Read the model definition and answer for the solid it produces. Units are mm, in the model's axes. A direction names the side the tool comes from. Coordinates: 2 decimals unless noted, no trailing zeros. Write each loop counter-clockwise with the first axis right and the second up, starting at its lowest first coordinate (ties: lowest second). Pieces come first, ordered by that corner, then holes.
Item 1: Straight lines are drawn through the part: probe 1 along Z at (x, y) = (-104, -100) (3 decimals); probe 2 along Z at (x, y) = (92, -38.5) (3 decimals); probe 3 along Y at (x, z) = (76.5, 61.5) (3 decimals). For each, find the intervals that lie inside material, in ascending order.
Item 2: Section A-A (x = -60) is taken. Give the vertices of the cut face in (y, z) (3 decimals), then the cut area to 3 significant figures.
Item 3: Section C-C (y = -89) is taken. Give the vertices of the cut face in (x, z) (3 decimals), then the cut area to 3 significant figures.
Item 4: Section B-B (z = 120.5) is taken. Give the vertices of the cut face in (x, y) (3 decimals), then the cut area to 3 significant figures.
Item 5: A tool of negligible diameter and unlimited length cuts with its end or side. For faces 1 (the face through (114.3, -4, 2)), 2 (the face through (-2, 5, 3.175)), from which of +Z, -Z, +X, -X, +Y, -Y can it reach the whole face along a straight path? Write none if from no direction.
Item 6: Determine the mould class of faces 3 (the face through (-101.62, -99.99, 102.13)), 4 (the face through (-102, -100, 27.4)), 5 (the face through (-2, 3, 0)), 6 (the face through (112.39, 99.79, 1.61)) for opening direction Z: released by +Z, released by -Z, zero draft, split by the parting line, or undercut.
Item 7: Each of these flat-tipped pins is pushed along its axis until it touches: P1, Ø8, axis at x = -88.5, y = -28.5, coming from the +Z side (3 decimals); P2, Ø1.5, axis at x = -44, z = 45.5, coming from the +Y side (3 decimals). Where does it stop, or does it pass through?
from build123d import *

# Parameters (mm, degrees)
SKETCH2_W           = 228.6
SKETCH2_H           = 203.2
BOSS_EXTRUDE1_DEPTH = 3.175
SKETCH3_W           = 228.6
SKETCH3_H           = 3.175
BOSS_EXTRUDE2_DEPTH = 127
FILLET1_R           = 3.175
FILLET2_R           = 6.35
SKETCH4_R           = 2.54
SKETCH4_R_2         = 2.15
SKETCH4_R_3         = 3.175
CUT_EXTRUDE1_DEPTH  = 265.612965007


with BuildPart() as part:
    # Sketch2 → Boss-Extrude1 (new body)
    with BuildSketch(Plane.XY):
        Rectangle(SKETCH2_W, SKETCH2_H)
    extrude(amount=BOSS_EXTRUDE1_DEPTH)

    # Sketch3 → Boss-Extrude2 (add)
    with BuildSketch(Plane.XY.offset(3.175)):
        with Locations((0, -100.0125)):
            Rectangle(SKETCH3_W, SKETCH3_H)
    extrude(amount=BOSS_EXTRUDE2_DEPTH)

    # Fillet1
    fillet1_edges = [part.edges().sort_by_distance(p)[0] for p in [
        (0, -98.425, 3.175),
        (0, -101.6, 0),
    ]]
    fillet(fillet1_edges, radius=FILLET1_R)

    # Fillet2
    fillet2_edges = [part.edges().sort_by_distance(p)[0] for p in [
        (-114.3, -100.0125, 130.175),
        (114.3, -100.0125, 130.175),
        (-114.3, 101.6, 1.5875),
        (114.3, 101.6, 1.5875),
    ]]
    fillet(fillet2_edges, radius=FILLET2_R)

    # Sketch4 → Cut-Extrude1 (cut, through all)
    with BuildSketch(Plane(origin=(0, -98.425, 0), x_dir=(1, 0, 0), z_dir=(0, 1, 0))):
        with Locations(Location((-104.14, -26.035, 0), (0, 0, 270))):
            Circle(SKETCH4_R)
        with Locations(Location((-104.14, -102.4636, 0), (0, 0, 270))):
            Circle(SKETCH4_R)
        with Locations(Location((0.4826, -26.035, 0), (0, 0, 270))):
            Circle(SKETCH4_R)
        with Locations(Location((-27.8257, -102.4636, 0), (0, 0, 270))):
            Circle(SKETCH4_R)
        with Locations(Location((68.25, -79.2493, 0), (0, 0, 270))):
            Circle(SKETCH4_R_2)
        with Locations(Location((97.95, -79.2493, 0), (0, 0, 270))):
            Circle(SKETCH4_R_2)
        with Locations(Location((68.25, -49.2493, 0), (0, 0, 270))):
            Circle(SKETCH4_R_2)
        with Locations(Location((97.95, -49.2493, 0), (0, 0, 270))):
            Circle(SKETCH4_R_2)
        with Locations(Location((-65.9257, -64.2493, 0), (0, 0, 270))):
            Circle(SKETCH4_R_3)
    extrude(amount=-CUT_EXTRUDE1_DEPTH, mode=Mode.SUBTRACT)


solid = part.part
Established:
1. probe 1: z = 0.418 to 23.499, 28.571 to 99.927, 105 to 130.175
1. probe 2: z = 0 to 3.175
1. probe 3: y = -101.6 to -98.425
2. outline: (-101.6, 3.175) arc R3.175 ccw to (-98.425, 0) - (101.6, 0) - (101.6, 3.175) - (-95.25, 3.175) arc R3.175 cw to (-98.425, 6.35) - (-98.425, 130.175) - (-101.6, 130.175) - close
2. area: 1,050 mm2
3. outline: (-114.3, 0) - (114.3, 0) - (114.3, 3.175) - (-114.3, 3.175) - close
3. area: 726 mm2
4. outline: (-114.3, -101.6) - (114.3, -101.6) - (114.3, -98.425) - (-114.3, -98.425) - close
4. area: 726 mm2
5. face 1: +Z, -Z, +X, +Y, -Y
5. face 2: +Z, +X, -X, +Y
6. face 3: undercut
6. face 4: undercut
6. face 5: released by -Z
6. face 6: zero draft
7. P1: stops at z = 3.175
7. P2: stops at y = -98.425
